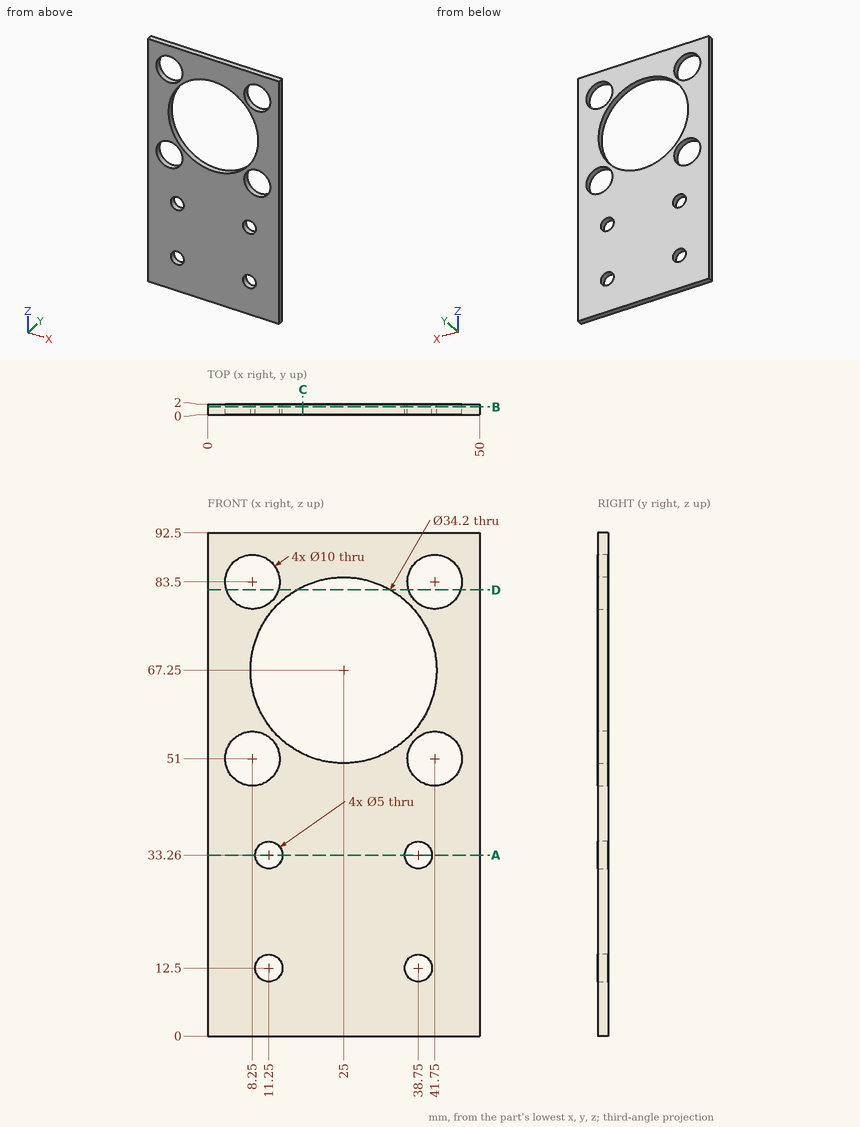
Job drawing, mm, ordinate dimensions from the low corner. One solid piece. Coordinates: 2 decimals unless noted, no trailing zeros. Order: outer loops, then holes, each group sorted by start corner. A loop starts at its lowest first (then second) coordinate and runs counter-clockwise, first axis right, second up. Notation, with made-up numbers: (-6.5, -4) - (8.5, -4) arc R11 ccw to (8.5, 9) - close; hole circle Ø1 at (39.5, 74.5). An arc over 180 degrees is marked (long way). Return JSON: item names as keys, results as strings. Group by question number.
1) Saw through at B-B, the plane y = 1.45. Count the separate pieces of the cut face and the enclosed holes in it, plus the area to 3 significant figures.
2) Saw through at D-D, the plane z = 82. Write the cut outline in (x, y).
3) Probe line 1 (X direction, y = 1.15, z = 33.26); line 2 (X direction, y = 1.5, z = 66.5); line 3 (X direction, y = 0.85, z = 47). List the from-to ranges inside material, lowest first. Write a range as from..to.
4) Saw through at A-A, the plane z = 33.26. Write the cut outline in (x, y), plus the area to 3 significant figures.
5) Flat gauge pin, fed straight in: P1, Ø6, axis at x = 41.75, z = 83.5, coming from the -Y side. Where does the tip first touch, or does it go through?
6) Saw through at C-C, the plane x = 17.5. Write the cut outline in (y, z).
Values found:
{
 "1": {"separate pieces": "1", "enclosed holes": "9", "area": "3,310 mm²"},
 "2": {"outline": "(0, 0) - (3.48, 0) - (3.48, 2) - (0, 2) - close; (13.02, 0) - (16.35, 0) - (16.35, 2) - (13.02, 2) - close; (33.65, 0) - (36.98, 0) - (36.98, 2) - (33.65, 2) - close; (46.52, 0) - (50, 0) - (50, 2) - (46.52, 2) - close"},
 "3": {"line 1": "x = 0..8.75, 13.75..36.25, 41.25..50", "line 2": "x = 0..7.92, 42.08..50", "line 3": "x = 0..5.25, 11.25..38.75, 44.75..50"},
 "4": {"outline": "(0, 0) - (8.75, 0) - (8.75, 2) - (0, 2) - close; (13.75, 0) - (36.25, 0) - (36.25, 2) - (13.75, 2) - close; (41.25, 0) - (50, 0) - (50, 2) - (41.25, 2) - close", "area": "80.0 mm²"},
 "5": {"P1": "passes through"},
 "6": {"outline": "(0, 0) - (2, 0) - (2, 51.88) - (0, 51.88) - close; (0, 82.62) - (2, 82.62) - (2, 92.5) - (0, 92.5) - close"}
}
